Autodesk Inventor part; units mm, degrees
ref_plane "YZ Plane" through (0, 0, 0) normal (1, 0, 0) x (0, 1, 0)
ref_plane "XZ Plane" through (0, 0, 0) normal (0, 1, 0) x (-1, 0, 0)
ref_plane "XY Plane" through (0, 0, 0) normal (0, 0, 1) x (1, 0, 0)
sketch "Sketch1" plane through (0, 0, 0) normal (0, 1, 0) x (-1, 0, 0)
  line L0 (-80.645, 0) -> (80.645, 0)
  line L1 (80.645, 0) -> (80.645, 12.7)
  line L2 (80.645, 12.7) -> (-80.645, 12.7)
  line L3 (-80.645, 12.7) -> (-80.645, 0)
  line L4 (-80.645, 0) -> (80.645, 12.7) construction
  line L5 (80.645, 0) -> (-80.645, 12.7) construction
  point P0 (0, 0)
  point P1 (0, 6.35)
  point P2 (0, 0)
  dimension "d0" = 12.7
  dimension "d1" = 161.29
extrude "Plate1" add sketch "Sketch1" along normal blind 0.9144
sketch "Sketch2" plane through (80.645, 0.0479, 11.7869) normal (0, -0.052336, 0.9986295) x (1, 0, 0)
  line L0 (-161.29, 0) -> (0, 0)
  line L1 (0, 0) -> (0, 12.7)
  line L2 (0, 12.7) -> (-161.29, 12.7)
  line L3 (-161.29, 12.7) -> (-161.29, 0)
edge flange "Flange1" height 12.7 angle 87 thickness 0.9144 bend radius 0.762 thickness toward (0, -0.052336, 0.9986295) relief tear relief width 0.9144 relief depth 0.4572 edges at (0, 0.9144, 12.7) wall of the first edge with corners at (-80.645, 0.0479, 11.7869) (80.645, 0.0479, 11.7869) (80.645, 12.7305, 12.4515) (-80.645, 12.7305, 12.4515)
bend "Bend1"
corner "Corner1"
sketch "Sketch3" plane through (0, 0.9144, 0) normal (0, 1, 0) x (1, 0, 0)
  line L0 (76.2, -3.81) -> (-76.2, -3.81) construction
  line L1 (-80.645, 0) -> (80.645, 0) construction
  point P0 (0, 0)
  point P1 (0, -3.81)
  point P2 (0, -3.81)
  point P3 (0, 0)
  dimension "d13" = 152.4
  dimension "d14" = 3.81
hole "Hole1" at (76.2, 0.9144, 3.81) at (0, 0.9144, 3.81) at (-76.2, 0.9144, 3.81) direction (0, -1, 0) diameter 3.2512 end through all
sketch "Sketch4" plane through (80.645, 12.7305, 12.4515) normal (0, 0.052336, -0.9986295) x (-1, 0, 0)
  line L0 (7.62, -3.81) -> (153.67, -3.81) construction
  line L1 (161.29, 0) -> (0, 0) construction
  point P0 (80.645, -13.3647)
  point P1 (80.645, -3.81)
  point P2 (80.645, -3.81)
  dimension "d22" = 146.05
  dimension "d23" = 3.81
hole "Hole2" at (73.025, 8.9257, 12.2521) at (0, 8.9257, 12.2521) at (-73.025, 8.9257, 12.2521) direction (0, -0.052336, 0.9986295) diameter 3.2512 end through all
chamfer "Corner Chamfer1" distance 5.588 angle 60 2 edges at (-80.645, 12.7065, 12.9081) (80.645, 12.7065, 12.9081) measured on face at (-26.8817, 12.6985, 13.0603)
fillet "Corner Round1" radius 3.81 6 edges at (80.645, 0.4572, 0) (-80.645, 0.4572, 0) (-75.057, 12.7065, 12.9081) (75.057, 12.7065, 12.9081) (-80.645, 3.0411, 12.4015) (80.645, 3.0411, 12.4015)
equation "\"d20\" = Thickness"
equation "\"d29\" = Thickness"
equation "\"d2\" = Thickness"
equation "\"d3\" = BendReliefWidth"
equation "\"d4\" = BendReliefDepth"
equation "\"d5\" = MinimumRemnant"
equation "\"d6\" = TransitionRadius"
equation "\"d9\" = BendRadius"
equation "\"d10\" = CornerReliefSize"
equation "\"d11\" = GapSize"
equation "\"d12\" = JacobiRadiusSize"
equation "\"BendReliefWidth\" = Thickness"
equation "\"BendReliefDepth\" = 0.5 * Thickness"
equation "\"CornerReliefSize\" = 4 * Thickness"
equation "\"MinimumRemnant\" = 2 * Thickness"
equation "\"TransitionRadius\" = BendRadius"
equation "\"JacobiRadiusSize\" = BendRadius"
equation "\"GapSize\" = Thickness"
properties part number "J009835" material "STAINLESS STEEL, 316"
Read the model definition and answer for the solid it produces. Units are mm, in the model's axes. Give positions to 0.01 mm unless a question says otherwise; leave off trailing zeros. Order: outer loops, then holes, each group sorted by start corner. A loop starts at its lowest first (then second) coordinate and runs counter-clockwise, first axis right, second up.
(1) Straight lines are drawn through the part: L1, parallel to X at y = 0.4, z = 3.81 (3 decimals); L2, parallel to Z at x = 0, y = 0.7; L3, parallel to Y at x = -66, z = 0.5. For each, find the intervals that lie inside material, in ascending order.
(2) For a pull along Y with two mould halves and no side action, classify faces 1 (the flat face through (1, 0.914, 6)), 2 (the cylindrical face through (-79.499, 0.464, 1.086)), 3 (the flat face through (1.129, 7.213, 13.078)), 4 (the cylindrical face through (74.6, 8.5, 12.7)) as released by +Y, released by -Y, zero draft, split by the parting line, or undercut.
(3) Find section C-C (y = 5.5). Give the vertices of the cut face in (x, z).
(4) Given pin 1 (4 mm diameter, centred on x = -9, y = 5.5, fed in from +Z); pin 2 (1 mm diameter, centred on x = 1.5, z = 11, fed in from +Y); pin 3 (1 mm diameter, centred on x = -34, z = 2.5, fed in from +Y), each flat-ended and moving along its own axis, determine where each tip first touches the part or whether it passes through.
(5) Find section B-B (z = 7.75). Give the vertices of the cut face in (x, y) (3 decimals), plus the area to 3 significant figures.
(6) Find section A-A (x = -5). Give the vertices of the cut face in (y, z).
Result sheet:
1. L1: x = -80.645 to -77.826, -74.574 to -1.626, 1.626 to 74.574, 77.826 to 80.645
1. L2: z = 0 to 2.18, 5.44 to 12.47
1. L3: y = 0 to 0.91
2. face 1: released by +Y
2. face 2: zero draft
2. face 3: released by -Y
2. face 4: undercut
3. outline: (-79.24, 12.07) - (79.24, 12.07) - (79.21, 12.99) - (-79.21, 12.99) - close
4. pin 1: stops at z = 13.09
4. pin 2: stops at y = 1.02
4. pin 3: stops at y = 0.91
5. outline: (-80.645, 0) - (80.645, 0) - (80.645, 0.914) - (-80.645, 0.914) - close
5. area: 147 mm2
6. outline: (0, 0) - (0.91, 0) - (0.91, 11.11) arc R0.76 cw to (1.64, 11.87) - (12.73, 12.45) - (12.68, 13.36) - (1.59, 12.78) arc R1.68 ccw to (0, 11.11) - close
